The drawing under review shows one solid part. Ordinate dimensions are in mm from its lowest x, y, z. Give positions to 0.01 mm unless a question says otherwise; leave off trailing zeros. Loops run counter-clockwise (first coordinate to the right, second up) from the corner with the lowest first, then second, coordinate; pieces in that order, holes last. Notation, with made-up numbers: (-6.5, -32) - (14.5, -32) arc R18 ccw to (14.5, -2) - close; hole circle Ø8 at (35.25, 4). An arc over 180 degrees is marked (long way). One line per item, written item: value. Start each with the question number.
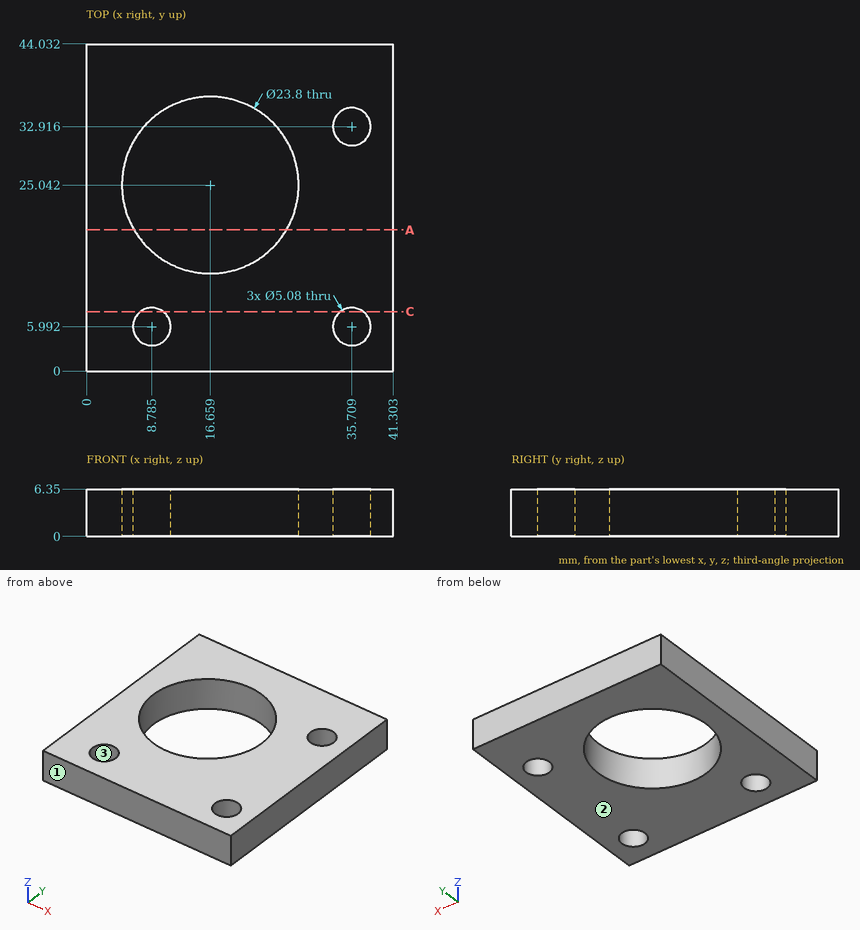
(1) To check wall thickness, follow L1, parallel to X at y = 6.5, z = 5; L2, parallel to X at y = 31.5, z = 3 (1 decimal); L3, parallel to Y at x = 7, z = 5 (1 decimal). State the ranges of each line that lie inside material, in increasing order. Write a range as from..to.
(2) Draft analysis for pull direction Y (two halves, no side actions). For the marked faces 1, 2 and 3, state which applies: pulls with the +Y half, pulls with the -Y half, needs draft (parallel to the pull), parting line crosses it, or undercut.
(3) Take a section at C-C on y = 8. State how many separate pieces and enclosed holes the cut face has, and give its area (3 significant figures).
(4) Take a section at A-A on y = 19. State the section outline as (x, z) points, and give its area (3 significant figures).
Here are the results:
1. L1: 0..6.3, 11.27..33.22, 38.2..41.3
1. L2: 0..6.7, 26.7..33.6, 37.8..41.3
1. L3: 0..4.2, 7.8..18.1, 32..44
2. face 1: pulls with the -Y half
2. face 2: needs draft
2. face 3: undercut
3. separate pieces: 3
3. enclosed holes: 0
3. area: 223 mm²
4. outline: (0, 0) - (6.41, 0) - (6.41, 6.35) - (0, 6.35) - close; (26.91, 0) - (41.3, 0) - (41.3, 6.35) - (26.91, 6.35) - close
4. area: 132 mm²
